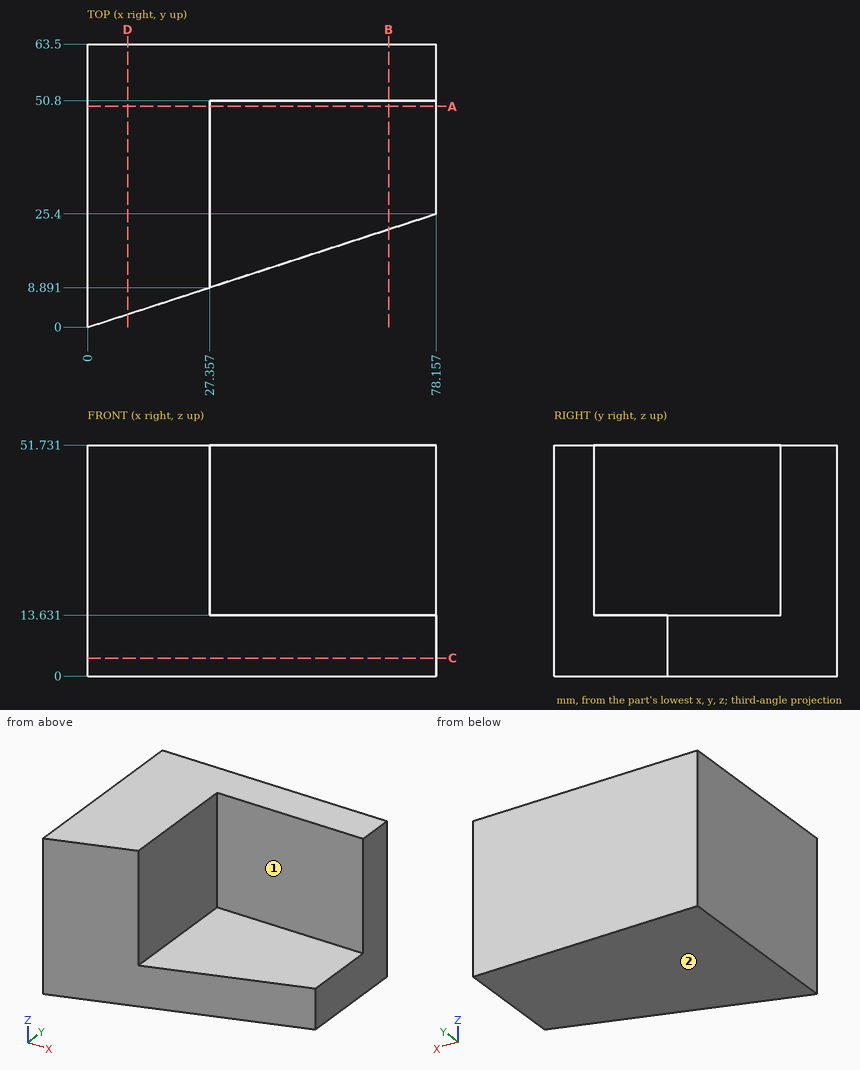
Could you check a few things on this drawing? It's one solid part, dimensions in mm from its lowest x, y, z. A direction names the side the tool comes from. Coordinates: 2 decimals unless noted, no trailing zeros. Write each loop counter-clockwise with the first axis right and the second up, starting at its lowest first coordinate (ties: lowest second). Pieces come first, ordered by that corner, then holes. Notation, with made-up numbers: (54, -26.5) - (66, -26.5) arc R8 cw to (66, -16.5) - close; hole circle Ø6 at (-26.75, -27). An arc over 180 degrees is marked (long way). Write item = value, one per line.
1) For the marked faces 1 and 2, which set-ups out of +Z, -Z, +X, -X, +Y, -Y let a thin tool reach every point of the face, with its end or its side?
Result set:
face_1 = +Z, +X, -Y
face_2 = -Z, +X, -X, +Y, -Y
2) Will these pins go through, and if not, where does the flat tip stop? pin 1 Ø8 at (x, z) = (46.5, 42) entering from -Y; pin 2 Ø1.5 at (x, y) = (28.5, 27) entering from +Z.
Result set:
pin_1 = 50.8
pin_2 = 13.63
3) Please list where these lines run through material, in increasing order: line 1 (X direction, y = 16.5, z = 35); line 2 (Y direction, x = 35.5, z = 37); line 3 (Z direction, x = 33, y = 50). Write a range as [from, to].
Result set:
line_1 = [0, 27.36]
line_2 = [50.8, 63.5]
line_3 = [0, 13.63]
4) Suppose I cut it at C-C on z = 4. Please give me the cut outline in (x, y).
Result set:
outline = (0, 0) - (78.16, 25.4) - (78.16, 63.5) - (0, 63.5) - close
5) Suppose I cut it at B-B on x = 67.5. Please give me the cut outline in (y, z), plus the area to 3 significant figures.
Result set:
outline = (21.94, 0) - (63.5, 0) - (63.5, 51.73) - (50.8, 51.73) - (50.8, 13.63) - (21.94, 13.63) - close
area = 1,050 mm2
6) Suppose I cut it at A-A on y = 49.5. Please give me the cut outline in (x, z), plus the area to 3 significant figures.
Result set:
outline = (0, 0) - (78.16, 0) - (78.16, 13.63) - (27.36, 13.63) - (27.36, 51.73) - (0, 51.73) - close
area = 2,110 mm2
7) Suppose I cut it at D-D on x = 9. Please give me the cut outline in (y, z) (1 decimal), plus the area to 3 significant figures.
Result set:
outline = (2.9, 0) - (63.5, 0) - (63.5, 51.7) - (2.9, 51.7) - close
area = 3,130 mm2
